For this review, take the finished solid that the model builds, in its own axes (mm). A direction names the side the tool comes from. Give positions to 0.01 mm unless a question says otherwise; leave off trailing zeros. Loops run counter-clockwise (first coordinate to the right, second up) from the corner with the lowest first, then second, coordinate; pieces in that order, holes last.
```python
from build123d import *

# Parameters (mm, degrees)
BOSS_EXTRUDE1_DEPTH = 0.79375
SKETCH2_W           = 6.35
SKETCH2_H           = 4.7625
CUT_EXTRUDE1_DEPTH  = 0.79375
SKETCH3_R           = 0.80645
SKETCH3_R_2         = 2.38125
CUT_EXTRUDE2_DEPTH  = 1.5875


with BuildPart() as part:
    # Sketch1 → Boss-Extrude1 (new body, symmetric)
    with BuildSketch(Plane(origin=(0, 0, 0), x_dir=(1, 0, 0), z_dir=(0, 1, 0))):
        Polygon((14.2875, 15.08125), (-14.2875, 15.08125), (-14.2875, -15.08125), (-7.9375, -15.08125), (-7.9375, 5.55625), (7.9375, 5.55625), (7.9375, -15.08125), (14.2875, -15.08125), align=None)
    extrude(amount=BOSS_EXTRUDE1_DEPTH, both=True)

    # Sketch2 → Cut-Extrude1 (cut)
    with BuildSketch(Plane(origin=(0, 0.79375, 0), x_dir=(1, 0, 0), z_dir=(0, 1, 0))):
        with Locations((-11.1125, -12.7)):
            Rectangle(SKETCH2_W, SKETCH2_H)
        with Locations((11.1125, -12.7)):
            Rectangle(SKETCH2_W, SKETCH2_H)
    extrude(amount=-CUT_EXTRUDE1_DEPTH, mode=Mode.SUBTRACT)

    # Sketch3 → Cut-Extrude2 (cut)
    with BuildSketch(Plane(origin=(0, 0.79375, 0), x_dir=(1, 0, 0), z_dir=(0, 1, 0))):
        with Locations((-11.1125, -12.7)):
            Circle(SKETCH3_R)
        with Locations((-7.9375, 10.31875)):
            Circle(SKETCH3_R_2)
        with Locations((11.1125, -12.7)):
            Circle(SKETCH3_R)
        with Locations((7.9375, 10.31875)):
            Circle(SKETCH3_R_2)
    extrude(amount=-CUT_EXTRUDE2_DEPTH, mode=Mode.SUBTRACT)


solid = part.part
```
Q1. For probe 1 along X at (y, z) = (-0.5, 12.7); probe 2 along X at (y, z) = (-0.2, 5); probe 3 along X at (y, z) = (-0.15, -10), list the stretches that pass through material, from the lowest coordinate up.
Answers:
probe 1: x = -14.29 to -11.92, -10.31 to -7.94, 7.94 to 10.31, 11.92 to 14.29
probe 2: x = -14.29 to -7.94, 7.94 to 14.29
probe 3: x = -14.29 to -10.3, -5.58 to 5.58, 10.3 to 14.29
Q2. Consider section C-C on z = 1.5. Give the boundary of the cut face in (x, y).
Answers:
outline: (-14.29, -0.79) - (-7.94, -0.79) - (-7.94, 0.79) - (-14.29, 0.79) - close; (7.94, -0.79) - (14.29, -0.79) - (14.29, 0.79) - (7.94, 0.79) - close
Q3. Consider section B-B on y = -0.5. Give the boundary of the cut face in (x, z), plus the area to 3 significant figures.
Answers:
outline: (-14.29, -15.08) - (14.29, -15.08) - (14.29, 15.08) - (7.94, 15.08) - (7.94, -5.56) - (-7.94, -5.56) - (-7.94, 15.08) - (-14.29, 15.08) - close; hole circle Ø1.61 at (-11.11, 12.7); hole circle Ø4.76 at (-7.94, -10.32); hole circle Ø4.76 at (7.94, -10.32); hole circle Ø1.61 at (11.11, 12.7)
area: 495 mm2
Q4. Consider section A-A on z = 12.7. Give the boundary of the cut face in (x, y), plus the area to 3 significant figures.
Answers:
outline: (-14.29, -0.79) - (-11.92, -0.79) - (-11.92, 0) - (-14.29, 0) - close; (-10.31, -0.79) - (-7.94, -0.79) - (-7.94, 0) - (-10.31, 0) - close; (7.94, -0.79) - (10.31, -0.79) - (10.31, 0) - (7.94, 0) - close; (11.92, -0.79) - (14.29, -0.79) - (14.29, 0) - (11.92, 0) - close
area: 7.52 mm2
Q5. For pin 1 Ø7.5 at (x, z) = (-7.94, -10.32) entering from -Y; pin 2 Ø2.5 at (x, z) = (-11.5, 12) entering from +Y; pin 3 Ø2 at (x, z) = (-6, 9) entering from +Y, all flat-tipped, find the tip position at first contact; note any pin that passes through.
Answers:
pin 1: stops at y = -0.79
pin 2: stops at y = 0
pin 3: passes through
Q6. Machinability: for faces 1 (the cylindrical face through (-10.316, 0.011, -10.423)), 2 (the flat face through (0, 0, -5.556)), 3 (the flat face through (10, 0, 13)), which of the approach directions +Z, -Z, +X, -X, +Y, -Y give a long, thin tool a straight path to every point of the face, cutting with its end or side? Answer none if there is none.
Answers:
face 1: +Y, -Y
face 2: +Z, +Y, -Y
face 3: +Z, +X, -X, +Y
Q7. Consider section D-D on x = 9.5. Give the boundary of the cut face in (y, z), plus the area to 3 significant figures.
Answers:
outline: (-0.79, -15.08) - (0.79, -15.08) - (0.79, -12.12) - (-0.79, -12.12) - close; (-0.79, -8.52) - (0.79, -8.52) - (0.79, 10.32) - (0, 10.32) - (0, 15.08) - (-0.79, 15.08) - close
area: 38.4 mm2
Q8. Mouldability with a two-part tool opening along X and no side actions: class faces 4 (the flat face through (14.288, 0, 0)), 5 (the flat face through (-7.938, 0, 5)), 6 (the flat face through (7.938, 0, 5)), 7 (the flat face through (0, 0.794, -8)) as +X half, -X half, draft (parallel to the pull), parting line (faces both ways), or undercut.
Answers:
face 4: +X half
face 5: undercut
face 6: undercut
face 7: draft
